```python
from build123d import *

# Parameters (mm, degrees)
F0_W      = 10
F0_H      = 12
F1_DEPTH  = 8
F2_W      = 10
F2_H      = 5.9
F3_DEPTH  = 15
F4_W      = 4
F4_H      = 5
F5_DEPTH  = 10
F7_DEPTH  = 25
F8_R      = 0.25
F9_R      = 1.25
F10_DEPTH = 4


with BuildPart() as f1:
    # F0 (on Top) → F1 (new body)
    with BuildSketch(Plane.XY):
        with Locations((5, 6)):
            Rectangle(F0_W, F0_H)
    extrude(amount=F1_DEPTH)

    # F2 (on face) → F3 (join)
    with BuildSketch(Plane.XY.offset(8)):
        with Locations((5, 2.95)):
            Rectangle(F2_W, F2_H)
    extrude(amount=F3_DEPTH)

    # F4 (on face) → F5 (cut, through all)
    with BuildSketch(Plane(origin=(0, 0, 0), x_dir=(0, -1, 0), z_dir=(-1, 0, 0))):
        Polygon((-1.9, 18), (-5.9, 18), (-5.9, 14), align=None)
        with Locations((-3.9, 20.5)):
            Rectangle(F4_W, F4_H)
        Polygon((-1.9, 23), (-1.9, 18), (0, 23), align=None)
    extrude(amount=-F5_DEPTH, mode=Mode.SUBTRACT)

    # F6 (on face) → F7 (cut)
    with BuildSketch(Plane.XZ):
        with BuildLine():
            ThreePointArc((2.25, 23), (5, 20.25), (7.75, 23))
            Line((7.75, 23), (2.25, 23))
        make_face()
    extrude(amount=-F7_DEPTH, mode=Mode.SUBTRACT)

    # F8
    f8_edges = [f1.edges().sort_by_distance(p)[0] for p in [
        (10, 6, 0),
        (10, 12, 4),
        (10, 8.95, 8),
        (10, 5.9, 11),
        (10, 3.9, 16),
        (10, 0.95, 20.5),
        (10, 0, 11.5),
        (0, 6, 0),
        (0, 0, 11.5),
        (0, 0.95, 20.5),
        (0, 3.9, 16),
        (0, 5.9, 11),
        (0, 8.95, 8),
        (0, 12, 4),
        (5, 12, 0),
        (5, 12, 8),
        (5, 0, 0),
    ]]
    fillet(f8_edges, radius=F8_R)

    # F9 (on face) → F10 (cut)
    with BuildSketch(Plane(origin=(0, 0, 0), x_dir=(1, 0, 0), z_dir=(0, 0, -1))):
        with Locations((5, -6)):
            Circle(F9_R)
    extrude(amount=-F10_DEPTH, mode=Mode.SUBTRACT)


solid = f1.part
```
Input: part model. Units: mm. Frame: model coordinates. A direction names the side the tool comes from. Give positions to 0.01 mm unless a question says otherwise; leave off trailing zeros. Write each loop counter-clockwise with the first axis right and the second up, starting at its lowest first coordinate (ties: lowest second). Pieces come first, ordered by that corner, then holes. Notation, with made-up numbers: (80, 55) - (129, 55) arc R9 cw to (129, 68) - close; hole circle Ø7 at (29.5, -15). An arc over 180 degrees is marked (long way). Write item = value, one per line. Start each with the question number.
1. Section query C-C, the plane z = 13.5. Output: boundary loops of the cut face in (x, y), then the cut area to 3 significant figures.
2. Section query B-B, the plane z = 3.5. Output: boundary loops of the cut face in (x, y).
3. Section query A-A, the plane x = 5. Output: boundary loops of the cut face in (y, z) (3 decimals), then the cut area to 3 significant figures.
4. First-contact query: pin 1 Ø4 at (x, y) = (8.5, 6.5) entering from +Z; pin 2 Ø3 at (x, z) = (5.5, 11.5) entering from +Y. Flat tips, straight axial feed; report the tip coordinate or a pass-through.
5. Section query D-D, the plane x = 1. Output: boundary loops of the cut face in (y, z), then the cut area to 3 significant figures.
6. Mould query, pull axis Y, two halves, no side actions, for faces 1 (the flat face through (5, 5.9, 11)), 2 (the cylindrical face through (4.73, 7.22, 1.97)), 3 (the flat face through (0, 5, 6)). Classes: released by +Y, released by -Y, zero draft, split by the parting line, or undercut.
7. Access query for faces 4 (the flat face through (5, 6, 4)), 5 (the flat face through (5, 9, 8)), 6 (the cylindrical face through (9.925, 3.802, 15.997)). Directions: +Z, -Z, +X, -X, +Y, -Y. A direction counts if a zero-diameter tool reaches every point of the face in a straight line with its end or side. Return the directions, or none.
8. Ray query, L1, parallel to X at y = 6, z = 1.4; L2, parallel to Y at x = 5, z = 2.7; L3, parallel to Z at x = 7.5, y = 6.5. Return the intervals inside material, ascending.
Check sheet entries:
q1.outline = (0, 0.25) arc R0.25 ccw to (0.25, 0) - (9.75, 0) arc R0.25 ccw to (10, 0.25) - (10, 5.65) arc R0.25 ccw to (9.75, 5.9) - (0.25, 5.9) arc R0.25 ccw to (0, 5.65) - close
q1.area = 58.9 mm2
q2.outline = (0, 0.25) arc R0.25 ccw to (0.25, 0) - (9.75, 0) arc R0.25 ccw to (10, 0.25) - (10, 11.75) arc R0.25 ccw to (9.75, 12) - (0.25, 12) arc R0.25 ccw to (0, 11.75) - close; hole circle Ø2.5 at (5, 6)
q3.outline = (0, 0.25) arc R0.25 ccw to (0.25, 0) - (4.75, 0) - (4.75, 4) - (7.25, 4) - (7.25, 0) - (11.75, 0) arc R0.25 ccw to (12, 0.25) - (12, 7.75) arc R0.25 ccw to (11.75, 8) - (5.9, 8) - (5.9, 14) - (1.9, 18) - (1.045, 20.25) - (0, 20.25) - close
q3.area = 140 mm2
q4.pin_1 = 15.4
q4.pin_2 = 5.9
q5.outline = (0, 0.25) arc R0.25 ccw to (0.25, 0) - (11.75, 0) arc R0.25 ccw to (12, 0.25) - (12, 7.75) arc R0.25 ccw to (11.75, 8) - (5.9, 8) - (5.9, 14) - (1.9, 18) - (0, 23) - close
q5.area = 152 mm2
q6.face_1 = released by +Y
q6.face_2 = undercut
q6.face_3 = zero draft
q7.face_4 = -Z
q7.face_5 = +Z, +X, -X, +Y
q7.face_6 = +Z, +X, +Y
q8.L1 = 0 to 3.75, 6.25 to 10
q8.L2 = 0 to 4.75, 7.25 to 12
q8.L3 = 0 to 8
